Print and shaded views of the part. All mm, measured from the part's lowest x, y and z. A direction names the side the tool comes from. Give positions to 0.01 mm unless a question says otherwise; leave off trailing zeros. Write each loop counter-clockwise with the first axis right and the second up, starting at its lowest first coordinate (ties: lowest second). Pieces come first, ordered by that corner, then holes. Notation, with made-up numbers: (81.5, 3) -> (138.5, 3) arc R31 ccw to (138.5, 34) -> close; hole circle Ø5 at (83.25, -36). An arc over 180 degrees is marked (long way). Put each result on its own line as item: value.
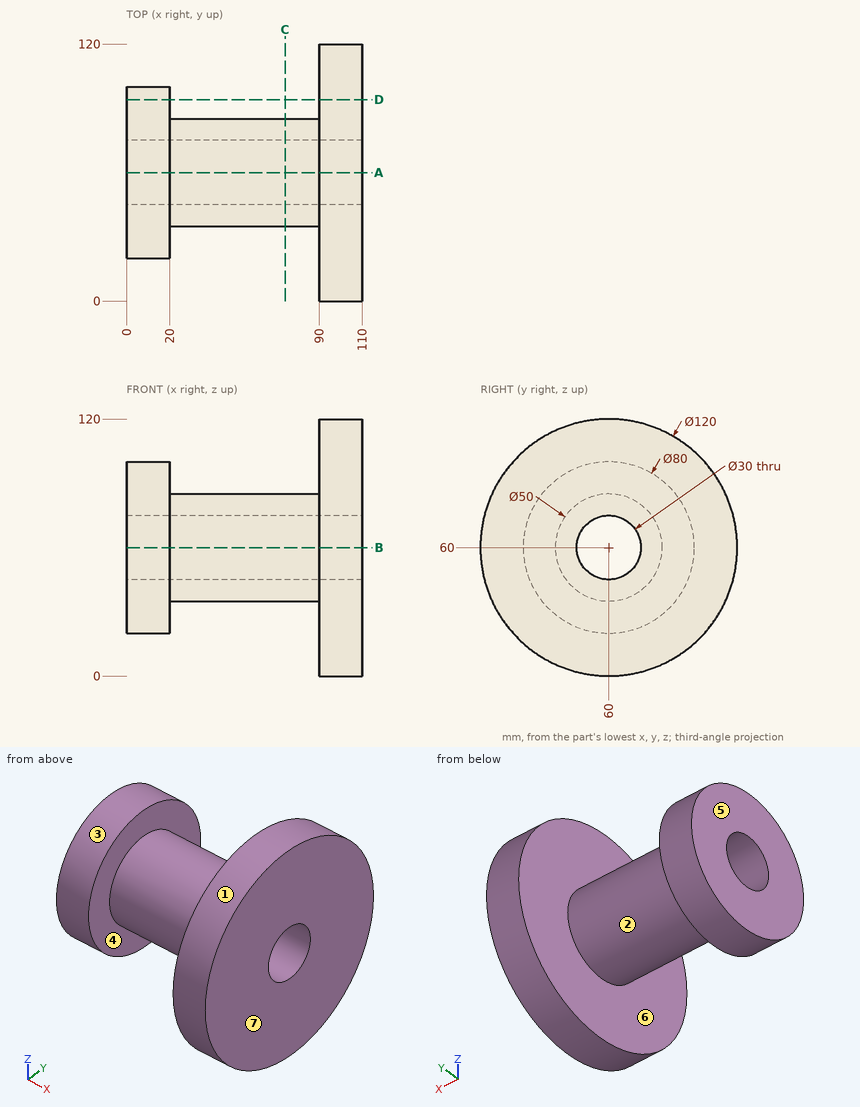
1) Pull direction X, two halves, no side cores. Call the marked faces 4, 5, 6 and 7: released by +X, released by -X, zero draft, split by the parting line, or undercut.
Filled sheet:
face 4: undercut
face 5: released by -X
face 6: undercut
face 7: released by +X
2) Slice it at A-A (y = 60). Write the cut outline in (x, z).
Filled sheet:
outline: (0, 20) -> (20, 20) -> (20, 35) -> (90, 35) -> (90, 0) -> (110, 0) -> (110, 45) -> (0, 45) -> close; (0, 75) -> (110, 75) -> (110, 120) -> (90, 120) -> (90, 85) -> (20, 85) -> (20, 100) -> (0, 100) -> close
3) Wall check: L1, parallel to X at y = 82.5, z = 87.5; L2, parallel to X at y = 98, z = 90; L3, parallel to Z at x = 71, y = 67. Give the ranges that are in metal, low to high.
Filled sheet:
L1: 0 to 20, 90 to 110
L2: 90 to 110
L3: 36 to 46.73, 73.27 to 84
4) Tool access for the marked faces 1, 2 and 3: list every direction of +Z, -Z, +X, -X, +Y, -Y with a clear straight run to the whole face (end or side of a thin tool).
Filled sheet:
face 1: +X, -X
face 2: none
face 3: -X
5) Slice it at D-D (y = 94). Write the cut outline in (x, z), plus the area to 3 significant figures.
Filled sheet:
outline: (0, 38.93) -> (20, 38.93) -> (20, 81.07) -> (0, 81.07) -> close; (90, 10.56) -> (110, 10.56) -> (110, 109.44) -> (90, 109.44) -> close
area: 2,820 mm2
6) Pin check, flat tips, straight feed: pin 1 (10 mm diameter, centred on x = 68.5, y = 40.5, fed in from -Z); pin 2 (1.5 mm diameter, centred on x = 66, y = 59, fed in from -Z); pin 3 (6 mm diameter, centred on x = 35.5, z = 76.5, fed in from -Y). Stop position of each tip, or through.
Filled sheet:
pin 1: z = 39.63
pin 2: z = 35
pin 3: y = 38.96
7) Slice it at C-C (x = 74). Write the cut outline in (y, z).
Filled sheet:
outline: circle Ø50 at (60, 60); hole circle Ø30 at (60, 60)
